Verification items for the finished model (mm, model axes). A direction names the side the tool comes from. Give positions to 0.01 mm unless a question says otherwise; leave off trailing zeros. Order: outer loops, then holes, each group sorted by start corner. A loop starts at its lowest first (then second) coordinate and runs counter-clockwise, first axis right, second up.
from build123d import *

# Parameters (mm, degrees)
SKETCH2_R          = 1.25
CUT_EXTRUDE1_DEPTH = 5.599304
CUT_EXTRUDE2_REACH = 8.599


with BuildPart() as part:
    # Sketch1 → Revolve1 (revolve)
    with BuildSketch(Plane(origin=(0, 0, 0), x_dir=(0, 0, -1), z_dir=(1, 0, 0))):
        with BuildLine():
            Line((0, 15.5), (20, 15.5))
            Line((20, 15.5), (20, 6.5))
            Line((20, 6.5), (26.2, 8))
            Line((26.2, 8), (26.2, 12.5))
            ThreePointArc((26.2, 12.5), (24.683117, 15.981117), (21.100696, 17.240231))
            Line((21.100696, 17.240231), (21.100696, 18.740231))
            ThreePointArc((21.100696, 18.740231), (25.744144, 17.041236), (27.7, 12.5))
            Line((27.7, 12.5), (27.7, 2.5))
            Line((27.7, 2.5), (20, 2.5))
            Line((20, 2.5), (18.05, 2.5))
            Line((18.05, 2.5), (18.05, 13.5))
            Line((18.05, 13.5), (1.95, 13.5))
            Line((1.95, 13.5), (1.95, 2.5))
            Line((1.95, 2.5), (0, 2.5))
            Line((0, 2.5), (0, 15.5))
        make_face()
    revolve(axis=Axis((0, 0, -20), (0, 0, 1)))

    # Sketch2 → Cut-Extrude1 (cut)
    with BuildSketch(Plane(origin=(0, 0, -27.7), x_dir=(-1, 0, 0), z_dir=(0, 0, -1))):
        with Locations((-6.717514, 6.717514)):
            Circle(SKETCH2_R)
        with Locations((6.717514, 6.717514)):
            Circle(SKETCH2_R)
        with Locations((6.717514, -6.717514)):
            Circle(SKETCH2_R)
        with Locations((-6.717514, -6.717514)):
            Circle(SKETCH2_R)
        with BuildLine():
            Line((-5.967514, 23.416114), (-5.967514, 12.717514))
            ThreePointArc((-5.967514, 12.717514), (-4.585786, 9.381728), (-1.25, 8))
            Line((-1.25, 8), (1.25, 8))
            ThreePointArc((1.25, 8), (4.585786, 9.381728), (5.967514, 12.717514))
            Line((5.967514, 12.717514), (5.967514, 23.416114))
            Line((5.967514, 23.416114), (-5.967514, 23.416114))
        make_face()
        with BuildLine():
            Line((-7.467514, 23.416114), (-7.467514, 10.279466))
            ThreePointArc((-7.467514, 10.279466), (-7.672459, 9.397549), (-8.245292, 8.696376))
            ThreePointArc((-8.245292, 8.696376), (-9.217507, 6.723535), (-8.254806, 4.746034))
            ThreePointArc((-8.254806, 4.746034), (-7.569897, 3.746571), (-7.587712, 2.53508))
            ThreePointArc((-7.587712, 2.53508), (-8, 0), (-7.587712, -2.53508))
            ThreePointArc((-7.587712, -2.53508), (-7.569897, -3.746571), (-8.254806, -4.746034))
            ThreePointArc((-8.254806, -4.746034), (-8.485281, -8.485281), (-4.746034, -8.254806))
            ThreePointArc((-4.746034, -8.254806), (-3.746571, -7.569897), (-2.53508, -7.587712))
            ThreePointArc((-2.53508, -7.587712), (0, -8), (2.53508, -7.587712))
            ThreePointArc((2.53508, -7.587712), (3.746571, -7.569897), (4.746034, -8.254806))
            ThreePointArc((4.746034, -8.254806), (8.485281, -8.485281), (8.254806, -4.746034))
            ThreePointArc((8.254806, -4.746034), (7.569897, -3.746571), (7.587712, -2.53508))
            ThreePointArc((7.587712, -2.53508), (8, 0), (7.587712, 2.53508))
            ThreePointArc((7.587712, 2.53508), (7.569897, 3.746571), (8.254806, 4.746034))
            ThreePointArc((8.254806, 4.746034), (9.217507, 6.723535), (8.245292, 8.696376))
            ThreePointArc((8.245292, 8.696376), (7.672459, 9.397549), (7.467514, 10.279466))
            Line((7.467514, 10.279466), (7.467514, 23.416114))
            ThreePointArc((7.467514, 23.416114), (0, -26.279016), (-7.467514, 23.416114))
        make_face()
    extrude(amount=-CUT_EXTRUDE1_DEPTH, mode=Mode.SUBTRACT)

    # Sketch3 → Cut-Extrude2 (cut, up to next)
    with BuildSketch(Plane.XY.offset(-21.100696), mode=Mode.PRIVATE) as cut_extrude2_sk1:
        with BuildLine():
            Line((7.467514, 17.1988), (7.467514, 15.502966))
            ThreePointArc((7.467514, 15.502966), (0, -17.207723), (-7.467514, 15.502966))
            Line((-7.467514, 15.502966), (-7.467514, 17.1988))
            ThreePointArc((-7.467514, 17.1988), (0, -18.75), (7.467514, 17.1988))
        make_face()
    cut_extrude2_tool1 = extrude(cut_extrude2_sk1.sketch, amount=-CUT_EXTRUDE2_REACH, mode=Mode.PRIVATE) & part.part
    add(cut_extrude2_tool1.solids().sort_by_distance((7.986992, 16.350883, -21.100696))[0], mode=Mode.SUBTRACT)


solid = part.part
(1) Scan lines: line 1 (Z direction, x = -7, y = 9.5); line 2 (Z direction, x = 11, y = 1); line 3 (X direction, y = 0, z = -0.8). Record each from-to range of solid material in increasing order.
Solved:
line 1: z = -27.7 to -26.2, -20 to -18.05, -1.95 to 0
line 2: z = -20 to -18.05, -1.95 to 0
line 3: x = -15.5 to -2.5, 2.5 to 15.5
(2) Section check B-B, the plane z = -24.5. Enter the section's corners in (x, y).
Solved:
outline: circle Ø15.18 at (0, 0); (-7.47, 14.31) arc R16.14 cw to (-5.97, 15) - (-5.97, 16.93) arc R17.96 ccw to (-7.47, 16.33) - close; (5.97, 15) arc R16.14 cw to (7.47, 14.31) - (7.47, 16.33) arc R17.96 ccw to (5.97, 16.93) - close; hole circle Ø5 at (0, 0)
(3) Section check A-A, the plane y = 0. Enter the section's corners in (x, z).
Solved:
outline: (-15.5, -20) - (-6.5, -20) - (-8, -26.2) - (-8, -27.7) - (-2.5, -27.7) - (-2.5, -18.05) - (-13.5, -18.05) - (-13.5, -1.95) - (-2.5, -1.95) - (-2.5, 0) - (-15.5, 0) - close; (2.5, -27.7) - (8, -27.7) - (8, -26.2) - (6.5, -20) - (15.5, -20) - (15.5, 0) - (2.5, 0) - (2.5, -1.95) - (13.5, -1.95) - (13.5, -18.05) - (2.5, -18.05) - close
(4) Section check D-D, the plane z = -7.5. Enter the section's corners in (x, y).
Solved:
outline: circle Ø31 at (0, 0); hole circle Ø27 at (0, 0)
(5) Go/stop test with flat-tipped pins: pin 1 (1 mm diameter, centred on x = 3, y = 17, fed in from +Z); pin 2 (4.5 mm diameter, centred on x = 0, y = 0, fed in from -Z); pin 3 (1.5 mm diameter, centred on x = -3, z = -12.5, fed in from -Y); pin 4 (5 mm diameter, centred on x = 1, z = -8.5, fed in from +Y). Record where each tip stops, or that it passes through.
Solved:
pin 1: stops at z = -21.1
pin 2: passes through
pin 3: stops at y = -15.34
pin 4: stops at y = 15.5
(6) Section check C-C, the plane x = -10. Enter the section's corners in (y, z).
Solved:
outline: (-11.84, -20) - (11.84, -20) - (11.84, 0) - (-11.84, 0) - close; hole (-9.07, -18.05) - (9.07, -18.05) - (9.07, -1.95) - (-9.07, -1.95) - close
(7) Release check for a two-part mould opening along X. For faces 1 (the flat face through (3, 0, 0)), 2 (the cylindrical face through (-7.565, 3.73, -26.96)), 3 (the cylindrical face through (2.44, -0.54, -0.96)) record: pulls with the +X half, pulls with the -X half, needs draft (parallel to the pull), parting line crosses it, or undercut.
Solved:
face 1: needs draft
face 2: pulls with the -X half
face 3: undercut
(8) Set-up check for faces 4 (the cylindrical face through (-7.678, 9.386, -26.958)), 5 (the cylindrical face through (3.763, -7.575, -26.96)), 6 (the flat face through (0, 8, -27)), 7 (the cylindrical face through (8, 0, -27)), 8 (the cylindrical face through (-6.555, 7.957, -26.96)): record each of +Z, -Z, +X, -X, +Y, -Y from which the full face is reachable in a straight line by a thin tool's end or side.
Solved:
face 4: -Z, -X, +Y
face 5: -Z, -Y
face 6: -Z, +Y
face 7: -Z, +X
face 8: -Z
